from build123d import *

# Parameters (mm, degrees)
MOTORPROFILE_W                                     = 56
MOTORPROFILE_H                                     = 58.42
BOSS_EXTRUDE2_DEPTH                                = 6.35
BOSS_EXTRUDE3_DEPTH                                = 64.77
CSK_FOR_10_FLAT_HEAD_MACHINE_SCREW_100_D           = 5.1054
CSK_FOR_10_FLAT_HEAD_MACHINE_SCREW_100_CSINK_D     = 9.779
CSK_FOR_10_FLAT_HEAD_MACHINE_SCREW_100_CSINK_ANGLE = 100


with BuildPart() as part:
    # MotorProfile → Boss-Extrude2 (new body)
    with BuildSketch(Plane(origin=(0, 0, 0), x_dir=(1, 0, 0), z_dir=(0, 1, 0))):
        Rectangle(MOTORPROFILE_W, MOTORPROFILE_H)
    extrude(amount=BOSS_EXTRUDE2_DEPTH)

    # Sketch2 → Boss-Extrude3 (add)
    with BuildSketch(Plane(origin=(0, 0, 0), x_dir=(1, 0, 0), z_dir=(0, 1, 0))):
        Polygon((-34.35, 29.21), (-34.35, -35.56), (28, -35.56), (28, -29.21), (-28, -29.21), (-28, 29.21), align=None)
    extrude(amount=BOSS_EXTRUDE3_DEPTH)

    # CSK for #10 Flat Head Machine Screw (100)1 (through all)
    with Locations(Plane(origin=(0, 6.35, 0), x_dir=(1, 0, 0), z_dir=(0, 1, 0))):
        with Locations((-17.960512242, 17.960512242), (-17.960512242, -17.960512242), (17.960512242, -17.960512242), (17.960512242, 17.960512242)):
            CounterSinkHole(CSK_FOR_10_FLAT_HEAD_MACHINE_SCREW_100_D / 2, CSK_FOR_10_FLAT_HEAD_MACHINE_SCREW_100_CSINK_D / 2, counter_sink_angle=CSK_FOR_10_FLAT_HEAD_MACHINE_SCREW_100_CSINK_ANGLE)


solid = part.part
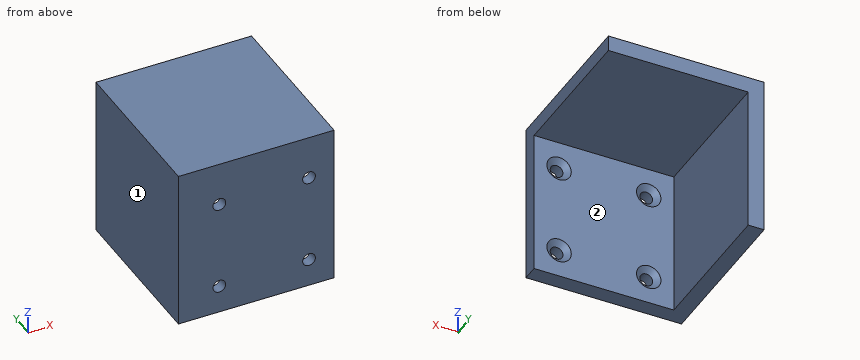
The listing builds one solid part. Answer for the finished solid, in the listing's coordinates (mm). Face numbers are marked on the shaded views. A direction names the side the tool comes from. Round coordinates to 2 decimals unless told otherwise and drop trailing zeros. Write each loop counter-clockwise with the first axis right and the second up, starting at its lowest first coordinate (ties: lowest second). Pieces come first, ordered by that corner, then holes. Notation, with made-up numbers: (23.25, 42) - (31.25, 42) arc R9 ccw to (31.25, 50) - close; hole circle Ø3 at (21.5, 41.25). An arc over 180 degrees is marked (long way). Use a Markdown table: item, result. Add a question column.
1. Flat-ended cylindrical pins translate along their axes: P1, Ø6.5, axis at x = -17.96, z = 17.96, coming from the -Y side; P2, Ø6.5, axis at x = -17.96, z = -17.96, coming from the +Y side; P3, Ø12, axis at x = -3.5, z = 0.5, coming from the +Y side; P4, Ø8, axis at x = -20, y = 10.5, coming from the -Z side. Find the tip coordinate at first contact, or state that the pin passes through.
2. The part is cut by section B-B (z = 7.5). Write down the section's boundary in (x, y), and give its area (3 significant figures).
3. The part is cut by section A-A (y = 49.5). Write down the section's boundary in (x, z).
4. A tool of negligible diameter and unlimited length cuts with its end or side. For the marked faces 1 and 2, from which of +Z, -Z, +X, -X, +Y, -Y can it reach the whole face along a straight path? Write none if from no direction.
5. Consider line 1 (Z direction, x = 6, y = 24); line 2 (X direction, y = 49, z = -25.5); line 3 (Y direction, x = 17.5, z = -7). Determine where each line is inside the solid, lowest interval first.
Reported:
| question | item | result |
|---|---|---|
| 1 | P1 | y = 0 |
| 1 | P2 | y = 4.97 |
| 1 | P3 | y = 6.35 |
| 1 | P4 | z = 29.21 |
| 2 | outline | (-34.35, 0) - (28, 0) - (28, 6.35) - (-28, 6.35) - (-28, 64.77) - (-34.35, 64.77) - close |
| 2 | area | 767 mm^2 |
| 3 | outline | (-34.35, -29.21) - (-28, -29.21) - (-28, 29.21) - (28, 29.21) - (28, 35.56) - (-34.35, 35.56) - close |
| 4 | face 1 | +Z, -Z, -X, +Y, -Y |
| 4 | face 2 | -Z, +X, +Y |
| 5 | line 1 | 29.21 to 35.56 |
| 5 | line 2 | -34.35 to -28 |
| 5 | line 3 | 0 to 6.35 |
